Could you check a few things on this model? Use its own coordinates, in mm. A direction names the side the tool comes from. Round coordinates to 2 decimals unless told otherwise and drop trailing zeros. Loops run counter-clockwise (first coordinate to the right, second up) from the corner with the lowest first, then second, coordinate; pieces in that order, holes last. Notation, with made-up numbers: (-39.75, 64.25) -> (-35.75, 64.25) arc R21 ccw to (-35.75, 80.25) -> close; hole circle Ø8 at (6.5, 51). An arc over 180 degrees is marked (long way). Write each question's results on one line, items separated by ' | '.
from build123d import *

# Parameters (mm, degrees)
SKETCH005_R     = 2
PAD003_DEPTH    = 5
PAD004_DEPTH    = 70
POCKET001_DEPTH = 70
FILLET017_R     = 2
FILLET018_R     = 1.9
FILLET019_R     = 1.9
FILLET020_R     = 1.9
FILLET021_R     = 1.89


with BuildPart() as part:
    # Sketch005 (on DatumPlane) → Pad003 (new body)
    with BuildSketch(Plane.XY.offset(58)):
        with BuildLine():
            Line((-33, 35), (33, 35))
            ThreePointArc((40, 28), (37.949747, 32.949747), (33, 35))
            Line((40, 28), (40, -28))
            ThreePointArc((33, -35), (37.949747, -32.949747), (40, -28))
            Line((33, -35), (-33, -35))
            ThreePointArc((-40, -28), (-37.949747, -32.949747), (-33, -35))
            Line((-40, -28), (-40, 28))
            ThreePointArc((-33, 35), (-37.949747, 32.949747), (-40, 28))
        make_face()
        with Locations((-25.5, 18.5)):
            Circle(SKETCH005_R, mode=Mode.SUBTRACT)
        with Locations((-25.5, -18.5)):
            Circle(SKETCH005_R, mode=Mode.SUBTRACT)
        with Locations((25.5, -18.5)):
            Circle(SKETCH005_R, mode=Mode.SUBTRACT)
        with Locations((25.5, 18.5)):
            Circle(SKETCH005_R, mode=Mode.SUBTRACT)
        with BuildLine():
            Line((28.5, 15.5), (28.5, -15.5))
            Line((25.5, -15.5), (28.5, -15.5))
            ThreePointArc((25.5, -15.5), (23.37868, -16.37868), (22.5, -18.5))
            Line((22.5, -18.5), (22.5, -21.5))
            Line((22.5, -21.5), (-22.5, -21.5))
            Line((-22.5, -18.5), (-22.5, -21.5))
            ThreePointArc((-22.5, -18.5), (-23.37868, -16.37868), (-25.5, -15.5))
            Line((-25.5, -15.5), (-28.5, -15.5))
            Line((-28.5, -15.5), (-28.5, 15.5))
            Line((-25.5, 15.5), (-28.5, 15.5))
            ThreePointArc((-25.5, 15.5), (-23.37868, 16.37868), (-22.5, 18.5))
            Line((-22.5, 18.5), (-22.5, 21.5))
            Line((-22.5, 21.5), (22.5, 21.5))
            Line((22.5, 21.5), (22.5, 18.5))
            ThreePointArc((22.5, 18.5), (23.37868, 16.37868), (25.5, 15.5))
            Line((25.5, 15.5), (28.5, 15.5))
        make_face(mode=Mode.SUBTRACT)
    extrude(amount=PAD003_DEPTH)

    # Sketch006 (on DatumPlane) → Pad004 (join)
    with BuildSketch(Plane.XY.offset(63)):
        with BuildLine():
            Line((20, 35), (33, 35))
            ThreePointArc((40, 28), (37.949747, 32.949747), (33, 35))
            Line((40, 28), (40, 26))
            Line((40, 26), (20, 26))
            Line((20, 26), (20, 35))
        make_face()
        with BuildLine():
            Line((-20, -26), (-40, -26))
            Line((-40, -26), (-40, -28))
            ThreePointArc((-40, -28), (-37.949747, -32.949747), (-33, -35))
            Line((-33, -35), (-20, -35))
            Line((-20, -35), (-20, -26))
        make_face()
        with BuildLine():
            Line((-20, 26), (-40, 26))
            Line((-40, 26), (-40, 28))
            ThreePointArc((-33, 35), (-37.949747, 32.949747), (-40, 28))
            Line((-33, 35), (-20, 35))
            Line((-20, 35), (-20, 26))
        make_face()
        with BuildLine():
            Line((27, -26), (40, -26))
            Line((40, -26), (40, -28))
            ThreePointArc((33, -35), (37.949747, -32.949747), (40, -28))
            Line((33, -35), (27, -35))
            Line((27, -35), (27, -26))
        make_face()
    extrude(amount=PAD004_DEPTH)

    # Sketch007 (on DatumPlane) → Pocket001 (cut)
    with BuildSketch(Plane.XY.offset(133)):
        with BuildLine():
            Line((21, 34), (33, 34))
            ThreePointArc((39, 28), (37.242641, 32.242641), (33, 34))
            Line((39, 28), (39, 27))
            Line((39, 27), (21, 27))
            Line((21, 27), (21, 34))
        make_face()
        with BuildLine():
            Line((-21, -27), (-39, -27))
            Line((-39, -27), (-39, -28))
            ThreePointArc((-39, -28), (-37.242641, -32.242641), (-33, -34))
            Line((-33, -34), (-21, -34))
            Line((-21, -34), (-21, -27))
        make_face()
        with BuildLine():
            Line((-21, 27), (-39, 27))
            Line((-39, 27), (-39, 28))
            ThreePointArc((-33, 34), (-37.242641, 32.242641), (-39, 28))
            Line((-33, 34), (-21, 34))
            Line((-21, 34), (-21, 27))
        make_face()
        with BuildLine():
            Line((28, -27), (39, -27))
            Line((39, -27), (39, -28))
            ThreePointArc((33, -34), (37.242641, -32.242641), (39, -28))
            Line((33, -34), (28, -34))
            Line((28, -34), (28, -27))
        make_face()
    extrude(amount=-POCKET001_DEPTH, mode=Mode.SUBTRACT)

    # Fillet017
    fillet017_edges = [part.edges().sort_by_distance(p)[0] for p in [
        (3.5, -35, 63),
    ]]
    fillet(fillet017_edges, radius=FILLET017_R)

    # Fillet018
    fillet018_edges = [part.edges().sort_by_distance(p)[0] for p in [
        (-20, -35, 98),
        (-20, -26, 98),
        (27, -35, 98),
        (27, -26, 98),
        (-40, -26, 98),
        (40, -26, 98),
    ]]
    fillet(fillet018_edges, radius=FILLET018_R)

    # Fillet019
    fillet019_edges = [part.edges().sort_by_distance(p)[0] for p in [
        (40, 0, 63),
        (-40, 0, 63),
    ]]
    fillet(fillet019_edges, radius=FILLET019_R)

    # Fillet020
    fillet020_edges = [part.edges().sort_by_distance(p)[0] for p in [
        (0, 35, 63),
    ]]
    fillet(fillet020_edges, radius=FILLET020_R)

    # Fillet021
    fillet021_edges = [part.edges().sort_by_distance(p)[0] for p in [
        (-40, 26, 98),
        (-20, 35, 98),
        (20, 35, 98),
        (20, 26, 98),
        (-20, 26, 98),
        (40, 26, 98),
    ]]
    fillet(fillet021_edges, radius=FILLET021_R)


solid = part.part
1) If we mould it in two halves opening along Y, with no side actions, what happens to faces 1 (the cylindrical face through (-38, -32.9, 95)), 2 (the flat face through (40, 0, 59)), 3 (the cylindrical face through (25.24, -16.517, 60.465))? For each: released by +Y, released by -Y, zero draft, split by the parting line, or undercut.
Model answer:
face 1: released by -Y | face 2: zero draft | face 3: undercut
2) I want a section at D-D, the plane z = 101. Give the number of separate pieces and of enclosed holes in the cut face, plus the area to 3 significant figures.
Model answer:
separate pieces: 4 | enclosed holes: 4 | area: 182 mm2
3) I want a section at B-B, the plane x = 5. Write out the boundary of the cut face in (y, z).
Model answer:
outline: (-35, 58) -> (-21.5, 58) -> (-21.5, 63) -> (-33, 63) arc R2 ccw to (-35, 61) -> close; (21.5, 58) -> (35, 58) -> (35, 61.1) arc R1.9 ccw to (33.1, 63) -> (21.5, 63) -> close
4) I want a section at A-A, the plane y = 6. Write out the boundary of the cut face in (x, z), plus the area to 3 significant figures.
Model answer:
outline: (-40, 58) -> (-28.5, 58) -> (-28.5, 63) -> (-38.1, 63) arc R1.9 ccw to (-40, 61.1) -> close; (28.5, 58) -> (40, 58) -> (40, 61.1) arc R1.9 ccw to (38.1, 63) -> (28.5, 63) -> close | area: 113 mm2
5) I need wall thicknesses on line 1 (Y direction, x = -26, z = 72); line 2 (Y direction, x = -25.5, z = 61.05); line 3 (X direction, y = -18, z = 59). Which ranges of each line are inside material? Lowest first, please.
Model answer:
line 1: y = -35 to -34, -27 to -26, 26 to 27, 34 to 35 | line 2: y = -35 to -20.5, -16.5 to -15.5, 15.5 to 16.5, 20.5 to 35 | line 3: x = -40 to -27.44, -23.56 to -22.54, 22.54 to 23.56, 27.44 to 40
6) I'm going to push flat-ended pins straight in: pin 1 (3.5 mm diameter, centred on y = 31.5, z = 98, fed in from -X); pin 2 (10 mm diameter, centred on x = -27.5, y = 13.5, fed in from +Z); pin 3 (2.5 mm diameter, centred on y = 31, z = 83, fed in from +X). Where does each tip first touch, or does it pass through?
Model answer:
pin 1: stops at x = -39.78 | pin 2: stops at z = 63 | pin 3: stops at x = 39.78
7) For faces 4 (the flat face through (-27, -34, 98)), 5 (the flat face through (28.5, 0, 60)), which set-ups out of +Z, -Z, +X, -X, +Y, -Y let a thin tool reach every point of the face, with its end or its side?
Model answer:
face 4: +Z | face 5: +Z, -Z
8) I want a section at C-C, the plane x = 30.5. Write out the boundary of the cut face in (y, z), plus the area to 3 significant figures.
Model answer:
outline: (-35, 58) -> (35, 58) -> (35, 133) -> (34, 133) -> (34, 63) -> (27, 63) -> (27, 133) -> (26, 133) -> (26, 63) -> (-26, 63) -> (-26, 133) -> (-27, 133) -> (-27, 63) -> (-34, 63) -> (-34, 133) -> (-35, 133) -> close | area: 630 mm2
